Read the model definition and answer for the solid it produces. Units are mm, in the model's axes. Face numbers are marked on the shaded views. Give positions to 0.01 mm unless a question says otherwise; leave off trailing zeros. Write each loop counter-clockwise with the first axis right and the second up, starting at its lowest first coordinate (ties: lowest second). Pieces come first, ordered by that corner, then holes. Notation, with made-up numbers: M 65.5,-23.75 L 78.5,-23.75 A22 cw 78.5,3.25 Z; hole C -5.75,86 d3. An arc over 180 degrees is marked long. Write each question's results on one line, items separated by ' | '. Start each with the question number.
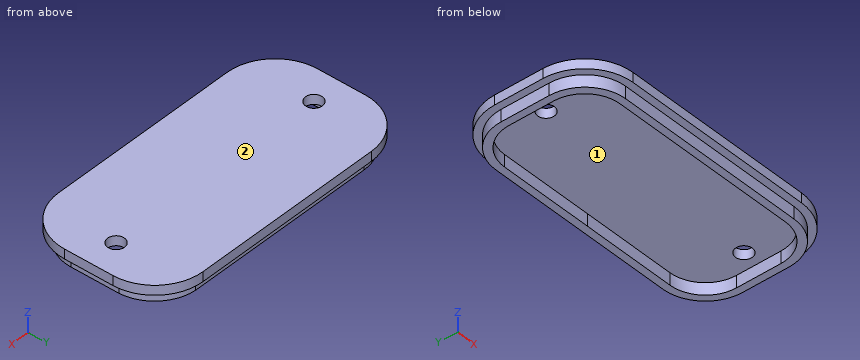
```python
from build123d import *

# Parameters (mm, degrees)
SKETCH_9_R      = 1.75
EXTRUDE_3_DEPTH = 2
EXTRUDE_START   = -2.5
EXTRUDE_4_DEPTH = 2.5


# Read off the part's stored shape, not the designer's step: Бобышка-Вытянуть4
with BuildPart() as part:
    # Эскиз9 → Бобышка-Вытянуть3 (new body)
    with BuildSketch(Plane.XY):
        with BuildLine():
            Line((-30, 8), (-30, -2))
            ThreePointArc((-30, -2), (-27.071067812, -9.071067812), (-20, -12))
            Line((-20, -12), (20, -12))
            ThreePointArc((20, -12), (27.071067812, -9.071067812), (30, -2))
            Line((30, -2), (30, 8))
            ThreePointArc((30, 8), (27.071067812, 15.071067812), (20, 18))
            Line((20, 18), (-20, 18))
            ThreePointArc((-20, 18), (-27.071067812, 15.071067812), (-30, 8))
        make_face()
        with Locations((23.5, 3)):
            Circle(SKETCH_9_R, mode=Mode.SUBTRACT)
        with Locations((-23.5, 3)):
            Circle(SKETCH_9_R, mode=Mode.SUBTRACT)
    extrude(amount=EXTRUDE_3_DEPTH)

    # Бобышка-Вытянуть4 outline → Бобышка-Вытянуть4 (add)
    with BuildSketch(Plane.XY.offset(EXTRUDE_START)):
        with BuildLine():
            Line((20, 16.5), (-20, 16.5))
            ThreePointArc((-20, 16.5), (-26.01040764, 14.01040764), (-28.5, 8))
            Line((-28.5, 8), (-28.5, -2))
            ThreePointArc((-28.5, -2), (-26.01040764, -8.01040764), (-20, -10.5))
            Line((-20, -10.5), (20, -10.5))
            ThreePointArc((20, -10.5), (26.01040764, -8.01040764), (28.5, -2))
            Line((28.5, -2), (28.5, 8))
            ThreePointArc((28.5, 8), (25.905867423, 13.905867423), (20, 16.5))
        make_face()
        with BuildLine():
            ThreePointArc((-19.623843683, -9.007966855), (-24.845207251, -6.845207251), (-27.007966855, -1.623843683))
            Line((-27.007966855, -1.623843683), (-27.007966855, 7.623843683))
            ThreePointArc((-27.007966855, 7.623843683), (-24.845207251, 12.845207251), (-19.623843683, 15.007966855))
            Line((-19.623843683, 15.007966855), (0, 15))
            Line((0, 15), (19.623843683, 15.007966855))
            ThreePointArc((19.623843683, 15.007966855), (24.845207251, 12.845207251), (27.007966855, 7.623843683))
            Line((27.007966855, 7.623843683), (27.007966855, -1.623843683))
            ThreePointArc((27.007966855, -1.623843683), (24.845207251, -6.845207251), (19.623843683, -9.007966855))
            Line((19.623843683, -9.007966855), (-19.623843683, -9.007966855))
        make_face(mode=Mode.SUBTRACT)
    extrude(amount=EXTRUDE_4_DEPTH)


solid = part.part
```
Item 1: Section A-A, the plane z = 0.95 is taken. Determine the outline of the cut face in (x, y), then the cut area to 3 significant figures.
Item 2: Section B-B, the plane y = 3 is taken. Determine the outline of the cut face in (x, z), then the cut area to 3 significant figures.
Item 3: Straight lines are drawn through the part: line 1 (X direction, y = 7, z = -0.3); line 2 (Y direction, x = 15, z = -2.3); line 3 (Z direction, x = -17, y = 5.5). For each, find the intervals that lie inside material, in ascending order.
Item 4: Determine the mould class of the marked faces 1 and 2 for opening direction Y: +Y half, -Y half, draft (parallel to the pull), parting line (faces both ways), or undercut.
Item 5: Section C-C, the plane x = 23.5 is taken. Determine the outline of the cut face in (y, z), then the cut area to 3 significant figures.
Item 6: Given P1, Ø7, axis at x = 4, y = 6.5, coming from the -Z side; P2, Ø2, axis at y = 3, z = -1.5, coming from the +X side; P3, Ø1.2, axis at x = 5.5, z = -1.5, coming from the -Y side; P4, Ø12, axis at x = -3.5, y = -5, coming from the -Z side, each flat-ended and moving along its own axis, determine where each tip first touches the part or whether it passes through.
Item 7: Section D-D, the plane y = 6 is taken. Determine the outline of the cut face in (x, z), then the cut area to 3 significant figures.
Worked out:
1) outline: M -30,-2 A10 ccw -20,-12 L 20,-12 A10 ccw 30,-2 L 30,8 A10 ccw 20,18 L -20,18 A10 ccw -30,8 Z; hole C -23.5,3 d3.5; hole C 23.5,3 d3.5 | area: 1,690 mm²
2) outline: M -30,0 L -28.5,0 L -28.5,-2.5 L -27.01,-2.5 L -27.01,0 L -25.25,0 L -25.25,2 L -30,2 Z; M -21.75,0 L 21.75,0 L 21.75,2 L -21.75,2 Z; M 25.25,0 L 27.01,0 L 27.01,-2.5 L 28.5,-2.5 L 28.5,0 L 30,0 L 30,2 L 25.25,2 Z | area: 113 mm²
3) line 1: x = -28.5 to -27.01, 27.01 to 28.5 | line 2: y = -10.5 to -9.01, 15.01 to 16.5 | line 3: z = 0 to 2
4) face 1: undercut | face 2: draft
5) outline: M -11.37,0 L -9.75,0 L -9.75,-2.5 L -7.91,-2.5 L -7.91,0 L 1.25,0 L 1.25,2 L -11.37,2 Z; M 4.75,0 L 13.91,0 L 13.91,-2.5 L 15.62,-2.5 L 15.62,0 L 17.37,0 L 17.37,2 L 4.75,2 Z | area: 59.3 mm²
6) P1: stops at z = 0 | P2: stops at x = 28.5 | P3: stops at y = -10.5 | P4: stops at z = -2.5
7) outline: M -30,0 L -28.5,0 L -28.5,-2.5 L -27.01,-2.5 L -27.01,0 L 27.01,0 L 27.01,-2.5 L 28.5,-2.5 L 28.5,0 L 30,0 L 30,2 L -30,2 Z | area: 127 mm²
